```python
from build123d import *

# Parameters (mm, degrees)
BOSS_EXTRUDE1_DEPTH = 6.35
SKETCH2_R           = 2.75
CUT_EXTRUDE1_DEPTH  = 7.35
FILLET1_R           = 15
CUT_EXTRUDE2_REACH  = 8.35
CUT_EXTRUDE3_REACH  = 8.35
SKETCH4_R           = 0.25


with BuildPart() as part:
    # Sketch1 → Boss-Extrude1 (new body)
    with BuildSketch(Plane(origin=(0, 0, 0), x_dir=(0, 0, -1), z_dir=(1, 0, 0))):
        with BuildLine():
            Line((-10, -22.912878475), (-10, -97.912878475))
            Line((-10, -97.912878475), (10, -97.912878475))
            Line((10, -97.912878475), (10, -22.912878475))
            ThreePointArc((10, -22.912878475), (0, 25), (-10, -22.912878475))
        make_face()
    extrude(amount=BOSS_EXTRUDE1_DEPTH)

    # Sketch2 → Cut-Extrude1 (cut, through all)
    with BuildSketch(Plane(origin=(6.35, 0, 0), x_dir=(0, 0, -1), z_dir=(1, 0, 0))):
        with Locations((0, -87.912878475)):
            Circle(SKETCH2_R)
        with Locations((0, -67.912878475)):
            Circle(SKETCH2_R)
        with Locations((0.431184648, -47.912878475)):
            Circle(SKETCH2_R)
    extrude(amount=-CUT_EXTRUDE1_DEPTH, mode=Mode.SUBTRACT)

    # Fillet1
    fillet1_edges = [part.edges().sort_by_distance(p)[0] for p in [
        (3.175, -22.912878475, 10),
        (3.175, -22.912878475, -10),
    ]]
    fillet(fillet1_edges, radius=FILLET1_R)

    # Sketch3 → Cut-Extrude2 (cut, up to next)
    with BuildSketch(Plane(origin=(6.35, 0, 0), x_dir=(0, 0, -1), z_dir=(1, 0, 0)), mode=Mode.PRIVATE) as cut_extrude2_sk1:
        Polygon((0, -7.505553499), (6.5, -3.75277675), (6.5, 3.75277675), (0, 7.505553499), (-6.5, 3.75277675), (-6.5, -3.75277675), align=None)
    cut_extrude2_tool1 = extrude(cut_extrude2_sk1.sketch, amount=-CUT_EXTRUDE2_REACH, mode=Mode.PRIVATE) & part.part
    add(cut_extrude2_tool1.solids().sort_by_distance((6.35, 0, 0))[0], mode=Mode.SUBTRACT)

    # Sketch4 → Cut-Extrude3 (cut, up to next)
    with BuildSketch(Plane(origin=(6.35, 0, 0), x_dir=(0, 0, -1), z_dir=(1, 0, 0)), mode=Mode.PRIVATE) as cut_extrude3_sk1:
        with Locations((0, 7.505553499)):
            Circle(SKETCH4_R)
    cut_extrude3_tool1 = extrude(cut_extrude3_sk1.sketch, amount=-CUT_EXTRUDE3_REACH, mode=Mode.PRIVATE) & part.part
    add(cut_extrude3_tool1.solids().sort_by_distance((6.35, 7.505553, 0))[0], mode=Mode.SUBTRACT)
    # Sketch4 → Cut-Extrude3 (cut, up to next)
    with BuildSketch(Plane(origin=(6.35, 0, 0), x_dir=(0, 0, -1), z_dir=(1, 0, 0)), mode=Mode.PRIVATE) as cut_extrude3_sk2:
        with Locations((6.5, 3.75277675)):
            Circle(SKETCH4_R)
    cut_extrude3_tool2 = extrude(cut_extrude3_sk2.sketch, amount=-CUT_EXTRUDE3_REACH, mode=Mode.PRIVATE) & part.part
    add(cut_extrude3_tool2.solids().sort_by_distance((6.35, 3.752777, -6.5))[0], mode=Mode.SUBTRACT)
    # Sketch4 → Cut-Extrude3 (cut, up to next)
    with BuildSketch(Plane(origin=(6.35, 0, 0), x_dir=(0, 0, -1), z_dir=(1, 0, 0)), mode=Mode.PRIVATE) as cut_extrude3_sk3:
        with Locations((6.5, -3.75277675)):
            Circle(SKETCH4_R)
    cut_extrude3_tool3 = extrude(cut_extrude3_sk3.sketch, amount=-CUT_EXTRUDE3_REACH, mode=Mode.PRIVATE) & part.part
    add(cut_extrude3_tool3.solids().sort_by_distance((6.35, -3.752777, -6.5))[0], mode=Mode.SUBTRACT)
    # Sketch4 → Cut-Extrude3 (cut, up to next)
    with BuildSketch(Plane(origin=(6.35, 0, 0), x_dir=(0, 0, -1), z_dir=(1, 0, 0)), mode=Mode.PRIVATE) as cut_extrude3_sk4:
        with Locations((0, -7.505553499)):
            Circle(SKETCH4_R)
    cut_extrude3_tool4 = extrude(cut_extrude3_sk4.sketch, amount=-CUT_EXTRUDE3_REACH, mode=Mode.PRIVATE) & part.part
    add(cut_extrude3_tool4.solids().sort_by_distance((6.35, -7.505553, 0))[0], mode=Mode.SUBTRACT)
    # Sketch4 → Cut-Extrude3 (cut, up to next)
    with BuildSketch(Plane(origin=(6.35, 0, 0), x_dir=(0, 0, -1), z_dir=(1, 0, 0)), mode=Mode.PRIVATE) as cut_extrude3_sk5:
        with Locations((-6.5, -3.75277675)):
            Circle(SKETCH4_R)
    cut_extrude3_tool5 = extrude(cut_extrude3_sk5.sketch, amount=-CUT_EXTRUDE3_REACH, mode=Mode.PRIVATE) & part.part
    add(cut_extrude3_tool5.solids().sort_by_distance((6.35, -3.752777, 6.5))[0], mode=Mode.SUBTRACT)
    # Sketch4 → Cut-Extrude3 (cut, up to next)
    with BuildSketch(Plane(origin=(6.35, 0, 0), x_dir=(0, 0, -1), z_dir=(1, 0, 0)), mode=Mode.PRIVATE) as cut_extrude3_sk6:
        with Locations((-6.5, 3.75277675)):
            Circle(SKETCH4_R)
    cut_extrude3_tool6 = extrude(cut_extrude3_sk6.sketch, amount=-CUT_EXTRUDE3_REACH, mode=Mode.PRIVATE) & part.part
    add(cut_extrude3_tool6.solids().sort_by_distance((6.35, 3.752777, 6.5))[0], mode=Mode.SUBTRACT)


solid = part.part
```
Work out the finished part from the listing and answer in its coordinate system (mm). A direction names the side the tool comes from. Round coordinates to 2 decimals unless told otherwise and drop trailing zeros. Loops run counter-clockwise (first coordinate to the right, second up) from the corner with the lowest first, then second, coordinate; pieces in that order, holes last. Notation, with made-up numbers: (-21, 50.5) -> (28, 50.5) arc R14 ccw to (28, 68.5) -> close; hole circle Ø7 at (-5, 9.25). An arc over 180 degrees is marked (long way). Write each question's results on one line, items separated by ' | '. Start each with the question number.
1. Section C-C (y = -16) is taken. Determine the outline of the cut face in (x, z), plus the area to 3 significant figures.
2. Section A-A (x = 2.5) is taken. State how many separate pieces and enclosed holes the cut face has, plus the area to 3 significant figures.
3. Find the intervals of material crossed by probe 1 along Y at (x, z) = (1.75, 0); probe 2 along Z at (x, y) = (4.5, -71); probe 3 along Z at (x, y) = (1.75, -68), in increasing order. Write a range as from..to.
4. Section B-B (z = 11.5) is taken. Determine the outline of the cut face in (x, y), plus the area to 3 significant figures.
5. Given pin 1 Ø1 at (x, y) = (5, -10.5) entering from +Z, flat-ended and moving along its own axis, determine where the tip first touches the part or whether it passes through.
6. A tool of negligible diameter and unlimited length cuts with its end or side. For faces 1 (the face through (3, -97.913, 0)), 2 (the face through (3, -64, 10)), 3 (the face through (3, 0, 6.5)), 4 (the face through (3, -65, -10)), from which of +Z, -Z, +X, -X, +Y, -Y can it reach the whole face along a straight path? Write none if from no direction.
Evaluation:
1) outline: (0, -19.21) -> (6.35, -19.21) -> (6.35, 19.21) -> (0, 19.21) -> close | area: 244 mm2
2) separate pieces: 1 | enclosed holes: 4 | area: 3,240 mm2
3) probe 1: y = -97.91..-90.66, -85.16..-70.66, -65.16..-50.63, -45.2..-7.76, 7.76..25 | probe 2: z = -10..10 | probe 3: z = -10..-2.75, 2.75..10
4) outline: (0, -24.69) -> (6.35, -24.69) -> (6.35, 22.2) -> (0, 22.2) -> close | area: 298 mm2
5) pin 1: stops at z = 22.91
6) face 1: +Z, -Z, +X, -X, -Y | face 2: +Z, +X, -X, -Y | face 3: +X, -X | face 4: -Z, +X, -X, -Y
